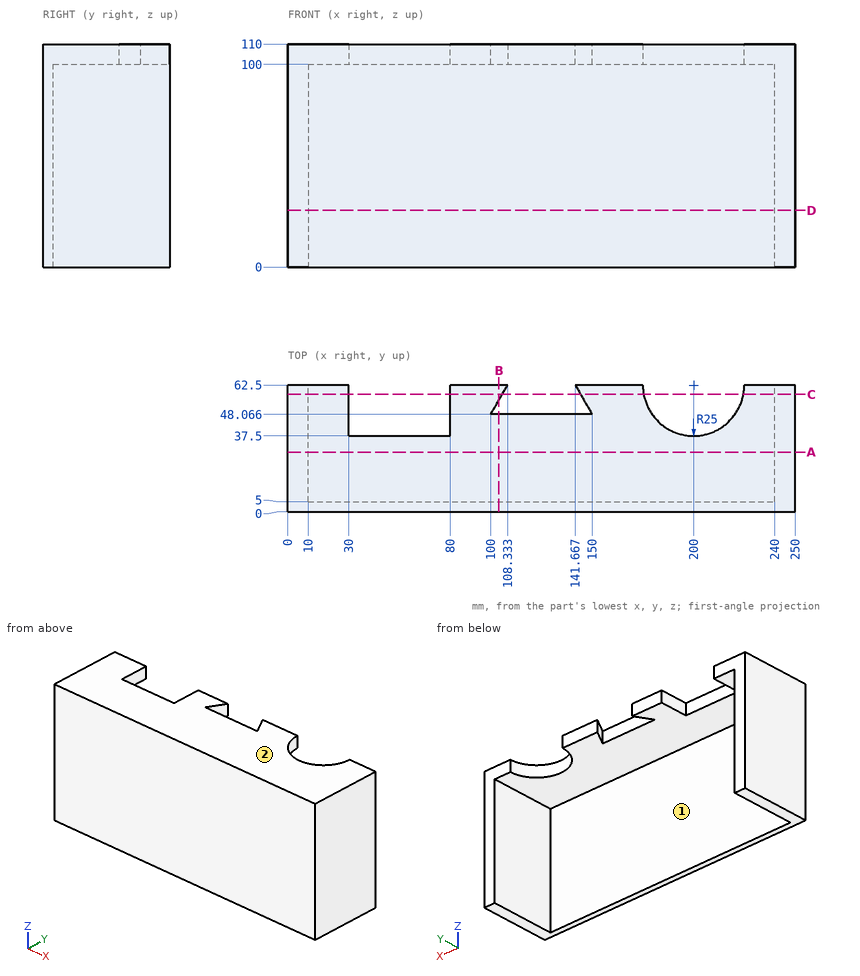
Input: dimensioned drawing with shaded views. Units: mm. Origin: part minimum x, y, z. A direction names the side the tool comes from. Round coordinates to 2 decimals unless told otherwise and drop trailing zeros. Order: outer loops, then holes, each group sorted by start corner. A loop starts at its lowest first (then second) coordinate and runs counter-clockwise, first axis right, second up. Notation, with made-up numbers: M 45.25,47 L 72.25,47 A22 cw 72.25,60 Z; hole C 45,-5 d6. An arc over 180 degrees is marked long. Use one line per item in the form item = value. Start each with the question number.
Q1. Material intervals for line 1 (X direction, y = 15, z = 28); line 2 (Y direction, x = 61, z = 63.5); line 3 (Z direction, x = 106.5, y = 48), sorted ascending. Write a range as [from, to].
Q2. Pin query (flat end, axial travel): pin 1 Ø5 at (x, z) = (48, 106.5) entering from +Y; pin 2 Ø2 at (x, z) = (138, 17.5) entering from +Y; pin 3 Ø11 at (x, z) = (133.5, 105.5) entering from +Y. Return the tip coordinate at first contact, or that it passes through.
Q3. Cut plane A-A (y = 29.5). Return loops of the section in (x, z), and give its area (3 significant figures).
Q4. Cut plane B-B (x = 104). Return loops of the section in (y, z) (1 decimal).
Q5. Access query for the marked faces 1 and 2. Directions: +Z, -Z, +X, -X, +Y, -Y. A direction counts if a zero-diameter tool reaches every point of the face in a straight line with its end or side. Return the directions, or none.
Q6. Cut plane C-C (y = 58). Return loops of the section in (x, z) (1 decimal), and give its area (3 significant figures).
Q7. Cut plane D-D (z = 28). Return loops of the section in (x, y).
Geometry results:
q1.line_1 = [0, 10], [240, 250]
q1.line_2 = [0, 5]
q1.line_3 = [100, 110]
q2.pin_1 = 37.5
q2.pin_2 = 5
q2.pin_3 = 48.07
q3.outline = M 0,0 L 10,0 L 10,100 L 240,100 L 240,0 L 250,0 L 250,110 L 0,110 Z
q3.area = 4,500 mm^2
q4.outline = M 0,0 L 5,0 L 5,100 L 48.1,100 L 48.1,110 L 0,110 Z; M 55,100 L 62.5,100 L 62.5,110 L 55,110 Z
q5.face_1 = -Z, +Y
q5.face_2 = +Z, +X, -X, +Y, -Y
q6.outline = M 0,0 L 10,0 L 10,100 L 30,100 L 30,110 L 0,110 Z; M 80,100 L 105.7,100 L 105.7,110 L 80,110 Z; M 144.3,100 L 175.4,100 L 175.4,110 L 144.3,110 Z; M 224.6,100 L 240,100 L 240,0 L 250,0 L 250,110 L 224.6,110 Z
q6.area = 3,120 mm^2
q7.outline = M 0,0 L 250,0 L 250,62.5 L 240,62.5 L 240,5 L 10,5 L 10,62.5 L 0,62.5 Z
